Could you check a few things on this model? Use its own coordinates, in mm. Face numbers are marked on the shaded views. A direction names the side the tool comes from. Coordinates: 2 decimals unless noted, no trailing zeros. Loops run counter-clockwise (first coordinate to the right, second up) from the corner with the lowest first, then second, coordinate; pieces in that order, holes last. Notation, with made-up numbers: (26, 35) - (36, 35) arc R20 ccw to (36, 48) - close; hole circle Ø1 at (49, -31). An arc over 180 degrees is marked (long way). One line per question, with ' | ' between items. Start each with the question number.
1. We'd pull the mould along X, two halves only. Please class the marked faces 4, 5 and 6: pulls with the +X half, pulls with the -X half, needs draft (parallel to the pull), parting line crosses it, or undercut.
2. I'm going to push flat-ended pins straight in: P1, Ø11, axis at y = -8.5, z = 4, coming from the +X side; P2, Ø4, axis at y = -6.5, z = 4.5, coming from the -X side; P3, Ø3, axis at x = 5, z = -7, coming from the -Y side; P4, Ø5, axis at y = -26, z = 3, coming from the -X side. Where does each tip first touch, or does it pass through?
3. Which directions (+Z, -Z, +X, -X, +Y, -Y) give clear straight access to the entire face, cutting with the end or side of a thin tool? Please do the marked faces 1, 2 and 3.
4. I want a section at A-A, the plane y = -27. Write out the boundary of the cut face in (x, z).
5. Please list where these lines run through material, in increasing order: L1, parallel to X at y = -4, z = 4.25; L2, parallel to X at y = -26, z = 7; L3, parallel to Y at x = 4.25, z = 10.25. Write a range as [from, to].
6. I want a section at B-B, the plane y = -21. Write out the boundary of the cut face in (x, z).
7. I want a section at C-C, the plane z = 3. Count the separate pieces of the cut face and the enclosed holes in it, then the cut area to 3 significant figures.
from build123d import *

# Parameters (mm, degrees)
LOFT_START                = -20
LOFT_2_DEPTH              = 20
SLOT_BOSS_EXTRUDE_DEPTH   = 3.5
NOTCH_CUT_EXTRUDE_DEPTH   = 4
F_6_0MM_DOWEL_HOLE1_D     = 6
CUT_EXTRUDE1_DEPTH        = 41.209626458
CUT_EXTRUDE1_DEPTH_BACK   = 41.209626458
F_2MM_DOWEL_HOLE_SKETCH_R = 1


# Read off the part's stored shape, not the designer's step: Loft
with BuildPart() as part:
    # Loft 2 outline → Loft 2 (new body)
    with BuildSketch(Plane(origin=(0, 0, 0), x_dir=(1.0, -2.490035096657917e-12, 0), z_dir=(2.490035096657917e-12, 1.0, -1.6178493389115347e-12)).offset(LOFT_START)):
        with BuildLine():
            add(Edge.make_bspline(
                [(-7.500000006, 10.153846153), (-6.876918809, 10.213864714), (-5.629329261, 10.319078273), (-3.754701534, 10.432067478), (-1.877896778, 10.499966465), (-0.625965179, 10.515066492), (0.625965179, 10.515066492), (1.877896376, 10.499966465), (3.754699934, 10.432067556), (5.629330497, 10.319078204), (6.876918808, 10.213864714), (7.5, 10.153846153)],
                knots=[0.804050837, 0.804050837, 0.804050837, 0.804050837, 0.828544483, 0.853038128, 0.877531773, 0.902025419, 0.902025419, 0.926519064, 0.951012709, 0.975506355, 1, 1, 1, 1], degree=3))
            add(Edge.make_bspline(
                [(-8.749999999, -11.846153861), (-8.82839887, -9.962671759), (-8.893913844, -6.220781941), (-8.718337998, -0.683170366), (-8.268913846, 4.779218054), (-7.786732208, 8.370661565), (-7.500000006, 10.153846153)],
                knots=[0.516152852, 0.516152852, 0.516152852, 0.516152852, 0.588127348, 0.660101844, 0.732076341, 0.804050837, 0.804050837, 0.804050837, 0.804050837], degree=3))
            Line((-8.749999999, -11.846153861), (8.75, -11.846153846))
            add(Edge.make_bspline(
                [(7.5, 10.153846153), (7.786732204, 8.370661588), (8.268913844, 4.779218073), (8.718337998, -0.683170354), (8.893913844, -6.220781934), (8.82839887, -9.962671757), (8.75, -11.846153846)],
                knots=[0, 0, 0, 0, 0.071974497, 0.143948993, 0.21592349, 0.287897986, 0.287897986, 0.287897986, 0.287897986], degree=3))
        make_face()
    extrude(amount=LOFT_2_DEPTH)

    # Slot Sketch → Slot Boss-Extrude (add, symmetric)
    with BuildSketch(Plane(origin=(0, 0, 0), x_dir=(0, 0, -1), z_dir=(1, 0, 0))):
        with BuildLine():
            Line((-11.846153846, -28.391743615), (-11.846153846, -12.033776613))
            ThreePointArc((-11.846153846, -12.033776613), (-2.846153846, -3.033776613), (6.153846154, -12.033776613))
            Line((6.153846154, -12.033776613), (6.153846154, -28.391743615))
            ThreePointArc((6.153846154, -28.391743615), (-2.846153846, -37.391743615), (-11.846153846, -28.391743615))
        make_face()
    extrude(amount=SLOT_BOSS_EXTRUDE_DEPTH, both=True)

    # Notch Sketch → Notch Cut-Extrude (cut, symmetric)
    with BuildSketch(Plane(origin=(0, 0, 0), x_dir=(0, 0, -1), z_dir=(1, 0, 0))):
        with BuildLine():
            Line((-15.97451802, -11.299393728), (-15.524991842, 1.708253078))
            Line((-15.524991842, 1.708253078), (11.860726968, 1.708253078))
            Line((11.860726968, 1.708253078), (11.18600525, -10.073329121))
            add(Edge.make_bspline(
                [(-15.97451802, -11.299393728), (-2.356980938, -16.766629454), (11.18600525, -10.073329121)],
                knots=[0, 0, 0, 1, 1, 1], degree=2))
        make_face()
    extrude(amount=NOTCH_CUT_EXTRUDE_DEPTH, both=True, mode=Mode.SUBTRACT)

    # Ø6.0mm Dowel Hole1 (through all)
    with Locations(Plane(origin=(3.5, 0, 0), x_dir=(0, 0, -1), z_dir=(1, 0, 0))):
        with Locations((-2.846153846, -28.391743615)):
            Hole(F_6_0MM_DOWEL_HOLE1_D / 2)

    # 2mm Dowel Hole Sketch → Cut-Extrude1 (cut, two sides: drawn at the far end of the back side and taken through both)
    with BuildSketch(Plane(origin=(0, 0, 0), x_dir=(0, 0, -1), z_dir=(1, 0, 0)).offset(-CUT_EXTRUDE1_DEPTH_BACK)):
        with Locations((-2.846153846, -4.070213016)):
            Circle(F_2MM_DOWEL_HOLE_SKETCH_R)
    extrude(amount=CUT_EXTRUDE1_DEPTH + CUT_EXTRUDE1_DEPTH_BACK, mode=Mode.SUBTRACT)


solid = part.part
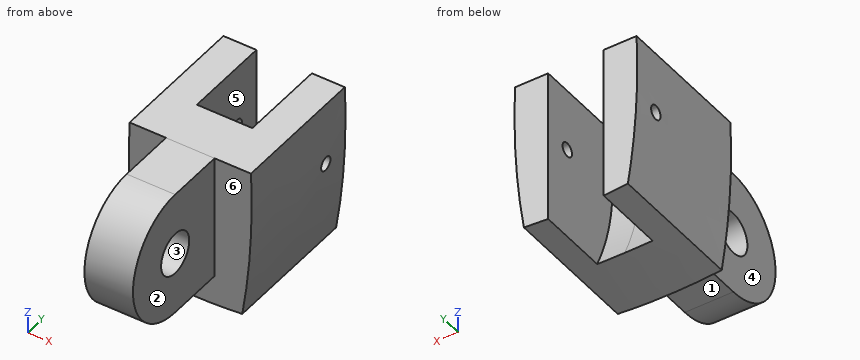
Results are:
1) face 4: pulls with the -X half | face 5: undercut | face 6: needs draft
2) P1: stops at x = 8.85 | P2: stops at x = -8.85 | P3: stops at y = -20 | P4: stops at x = -3.5
3) face 1: -Z, +X, -X, -Y | face 2: +Z, -Z, +X, -Y | face 3: +X, -X
4) outline: (-3.5, -6.15) - (3.5, -6.15) - (3.5, 0.19) - (-3.5, 0.19) - close; (-3.5, 5.5) - (3.5, 5.5) - (3.5, 11.85) - (-3.5, 11.85) - close
5) L1: x = [-8.82, -4], [4, 8.82] | L2: x = [-3.5, 3.5] | L3: y = [-20, 0]
6) outline: (-3.5, -6.15) - (3.5, -6.15) - (3.5, 11.85) - (-3.5, 11.85) - close
7) separate pieces: 4 | enclosed holes: 0 | area: 302 mm2
